Check sheet for the modelled part. Datum: model origin and axes. Units: mm. A direction names the side the tool comes from. Coordinates: 2 decimals unless noted, no trailing zeros. Loops run counter-clockwise (first coordinate to the right, second up) from the corner with the lowest first, then second, coordinate; pieces in that order, holes last. Notation, with made-up numbers: M 81.25,74 L 135.25,74 A9 ccw 135.25,91 Z; hole C 54.25,68.5 d8. An arc over 180 degrees is marked long. Use CSV: the item, a comma, the result in double quotes. Start each with the question number.
(1) Section check B-B on y = 48.5. Record the cut outline in (x, z), and give its area (3 significant figures).
(2) Draft check along X on faces 3 (the flat face through (-28.2, 0, 15.3)), 4 (the conical face through (-8.348, 42.285, -10.888)), 5 (the cylindrical face through (0.66, 48.944, -14.985)). Enter one of: pulls with the +X half, pulls with the -X half, needs draft (parallel to the pull), parting line crosses it, or undercut.
(3) Scan lines: line 1 (X direction, y = 46, z = 0); line 2 (X direction, y = 21.5, z = 0); line 3 (Z direction, x = -22.5, y = 25). Record each from-to range of solid material in increasing order.
(4) Section check A-A on z = 0. Record the cut outline in (x, y).
(5) Set-up check for faces 1 (the cylindrical face through (34.454, 17.255, -4.524)), 2 (the cylindrical face through (-30.995, 16.346, -6.883)): record each of +Z, -Z, +X, -X, +Y, -Y from which the full face is reachable in a straight line by a thin tool's end or side.
(6) Go/stop test with flat-tipped pins: pin 1 Ø4 at (x, z) = (2.5, -17) entering from -Y; pin 2 Ø6 at (x, y) = (-6.5, 14.5) entering from -Z; pin 3 Ø2 at (x, z) = (4.5, -26.5) entering from +Y. Record where each tip stops, or that it passes through.
(7) Section check C-C on y = 17.5. Record the cut outline in (x, z).
from build123d import *

# Parameters (mm, degrees)
SKETCH_1_R               = 34.75
EXTRUDE_1_DEPTH          = 35
SKETCH_2_R               = 15
EXTRUDE_2_DEPTH          = 8
SHELL_2_T                = -3
CUT_EXTRUDE_1_DEPTH      = 73.278108815
CUT_EXTRUDE_1_DEPTH_BACK = 73.278108815
SKETCH_3_R               = 12.8


with BuildPart() as part:
    # 스케치1 → 보스-돌출1 (new body)
    with BuildSketch(Plane(origin=(0, 0, 0), x_dir=(1, 0, 0), z_dir=(0, 1, 0))):
        with Locations(Location((0, 0, 0), (0, 0, 270))):
            Circle(SKETCH_1_R)
    extrude(amount=EXTRUDE_1_DEPTH)



with BuildPart() as body_2:
    # 스케치2 → 보스-돌출2 (new body)
    with BuildSketch(Plane(origin=(0, 45, 0), x_dir=(1, 0, 0), z_dir=(0, 1, 0))):
        with Locations(Location((0, 0, 0), (0, 0, 270))):
            Circle(SKETCH_2_R)
    extrude(amount=EXTRUDE_2_DEPTH)


with BuildPart() as part_1:
    add(part.part)

    add(body_2.part)  # loft_1 joins it to this body
    # loft from a face of the part (loft_1)
    loft([part_1.faces().sort_by_distance((0, 35, 0))[0], part_1.faces().sort_by_distance((0, 45, 0))[0]])

    # 쉘2
    shell_2_openings = [part_1.faces().sort_by_distance(p)[0] for p in [
        (0, 0, 0),
    ]]
    offset(amount=SHELL_2_T, openings=shell_2_openings, kind=Kind.INTERSECTION)

    # 스케치3 → 컷-돌출1 (cut, two sides: drawn at the far end of the back side and taken through both)
    with BuildSketch(Plane(origin=(0, 53, 0), x_dir=(1, 0, 0), z_dir=(0, 1, 0)).offset(-CUT_EXTRUDE_1_DEPTH_BACK)):
        with Locations(Location((0, 0, 0), (0, 0, 270))):
            Circle(SKETCH_3_R)
    extrude(amount=CUT_EXTRUDE_1_DEPTH + CUT_EXTRUDE_1_DEPTH_BACK, mode=Mode.SUBTRACT)


solid = part_1.part
Outcome:
1,outline,"C 0,0 d30; hole C 0,0 d25.6"
1,area,"192 mm²"
2,face 3,"needs draft"
2,face 4,"undercut"
2,face 5,"parting line crosses it"
3,line 1,"x = -15 to -12.8, 12.8 to 15"
3,line 2,"x = -34.75 to -31.75, 31.75 to 34.75"
3,line 3,"z = -26.48 to -22.4, 22.4 to 26.48"
4,outline,"M -34.75,0 L -31.75,0 L -31.75,33.16 L -12.8,42.75 L -12.8,53 L -15,53 L -15,45 L -34.75,35 Z; M 12.8,42.75 L 31.75,33.16 L 31.75,0 L 34.75,0 L 34.75,35 L 15,45 L 15,53 L 12.8,53 Z"
5,face 1,"+Y, -Y"
5,face 2,"-Y"
6,pin 1,"stops at y = 39.52"
6,pin 2,"stops at z = -34.57"
6,pin 3,"stops at y = 39.49"
7,outline,"C 0,0 d69.5; hole C 0,0 d63.5"
